The model under review builds one solid part; all positions refer to its coordinate system, in mm. Face numbers are marked on the shaded views. Round coordinates to 2 decimals unless told otherwise and drop trailing zeros. Loops run counter-clockwise (first coordinate to the right, second up) from the corner with the lowest first, then second, coordinate; pieces in that order, holes last. Notation, with made-up numbers: (-16.75, -27.5) -> (-7.75, -27.5) arc R24 cw to (-7.75, 0.5) -> close; hole circle Ø9 at (67.5, 84). An arc over 180 degrees is marked (long way). Return JSON: item names as keys, results as strings. Group by question number.
```python
from build123d import *

# Parameters (mm, degrees)
SKETCH_1_W          = 30
SKETCH_1_H          = 30
SKETCH_1_W_2        = 24
SKETCH_1_H_2        = 24
EXTRUDE_1_DEPTH     = 320
CUT_EXTRUDE_1_DEPTH = 323.800247831
SKETCH_3_R          = 2.1
CUT_EXTRUDE_2_DEPTH = 323.800247831
CUT_EXTRUDE_4_DEPTH = 323.800247831


with BuildPart() as part:
    # 草图1 → 拉伸-薄壁1 (new body)
    with BuildSketch(Plane.XY):
        with Locations((15, 15)):
            Rectangle(SKETCH_1_W, SKETCH_1_H)
        with Locations((15, 15)):
            Rectangle(SKETCH_1_W_2, SKETCH_1_H_2, mode=Mode.SUBTRACT)
    extrude(amount=EXTRUDE_1_DEPTH)

    # 草图2 → 切除-拉伸1 (cut, through all)
    with BuildSketch(Plane(origin=(30, 0, 0), x_dir=(0, 0, -1), z_dir=(1, 0, 0))):
        with BuildLine():
            Line((-277.5, 25), (-207.5, 25))
            ThreePointArc((-207.5, 25), (-197.5, 15), (-207.5, 5))
            Line((-207.5, 5), (-277.5, 5))
            ThreePointArc((-277.5, 5), (-287.5, 15), (-277.5, 25))
        make_face()
    extrude(amount=-CUT_EXTRUDE_1_DEPTH, mode=Mode.SUBTRACT)

    # 草图3 → 切除-拉伸2 (cut, through all)
    with BuildSketch(Plane(origin=(0, 30, 0), x_dir=(1, 0, 0), z_dir=(0, 1, 0))):
        with Locations(Location((15, -20, 0), (0, 0, 270))):
            Circle(SKETCH_3_R)
        with Locations(Location((15, -55, 0), (0, 0, 270))):
            Circle(SKETCH_3_R)
        with Locations(Location((15, -90, 0), (0, 0, 270))):
            Circle(SKETCH_3_R)
        with Locations(Location((15, -125, 0), (0, 0, 270))):
            Circle(SKETCH_3_R)
        with Locations(Location((15, -300, 0), (0, 0, 90))):
            Circle(SKETCH_3_R)
        with Locations(Location((15, -265, 0), (0, 0, 90))):
            Circle(SKETCH_3_R)
        with Locations(Location((15, -230, 0), (0, 0, 90))):
            Circle(SKETCH_3_R)
        with Locations(Location((15, -195, 0), (0, 0, 90))):
            Circle(SKETCH_3_R)
        with Locations(Location((15, -160, 0), (0, 0, 270))):
            Circle(SKETCH_3_R)
    extrude(amount=-CUT_EXTRUDE_2_DEPTH, mode=Mode.SUBTRACT)

    # 草图4 → 切除-拉伸4 (cut, through all)
    with BuildSketch(Plane(origin=(0, 0, 0), x_dir=(0, 0, -1), z_dir=(1, 0, 0))):
        Polygon((-180, 30), (-140, 3), (-80, 3), (-65, 30), align=None)
    extrude(amount=CUT_EXTRUDE_4_DEPTH, mode=Mode.SUBTRACT)


solid = part.part
```
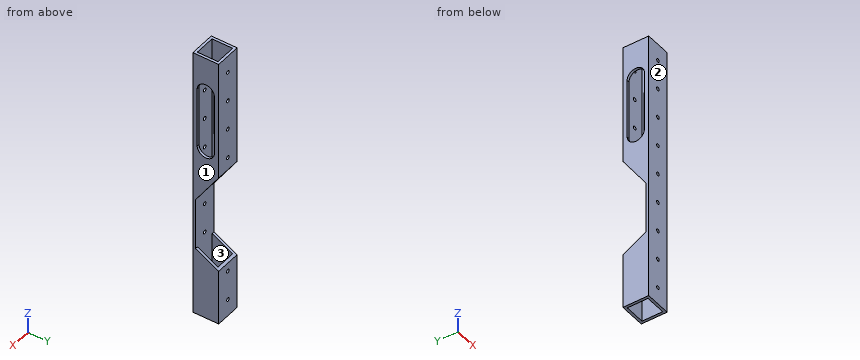
1. For P1, Ø6.5, axis at x = 15, z = 160, coming from the +Y side; P2, Ø5, axis at x = 15, z = 195, coming from the -Y side; P3, Ø2.5, axis at x = 15, z = 265, coming from the -Y side, all flat-tipped, find the tip position at first contact; note any pin that passes through.
2. Draft analysis for pull direction X (two halves, no side actions). For the marked faces 1, 2 and 3, state which applies: pulls with the +X half, pulls with the -X half, needs draft (parallel to the pull), parting line crosses it, or undercut.
3. We need section B-B, the plane z = 257. Write out the cut boundary in (x, y), then the cut area to 3 significant figures.
4. Wall thickness on line 1 (Y direction, x = 22, z = 291); line 2 (X direction, y = 28.1, z = 195): over which ranges is each line inside the solid? List them lowest first.
5. We need section A-A, the plane x = 21. Write out the cut boundary in (y, z).
6. We need section D-D, the plane z = 36.5. Write out the cut boundary in (x, y).
7. We need section C-C, the plane y = 22. Write out the cut boundary in (x, z), then the cut area to 3 significant figures.
Check sheet entries:
{
 "1": {"P1": "stops at y = 3", "P2": "stops at y = 0", "P3": "passes through"},
 "2": {"face 1": "pulls with the +X half", "face 2": "needs draft", "face 3": "undercut"},
 "3": {"outline": "(0, 0) -> (30, 0) -> (30, 5) -> (27, 5) -> (27, 3) -> (3, 3) -> (3, 5) -> (0, 5) -> close; (0, 25) -> (3, 25) -> (3, 27) -> (27, 27) -> (27, 25) -> (30, 25) -> (30, 30) -> (0, 30) -> close", "area": "204 mm²"},
 "4": {"line 1": "y = 0 to 3, 27 to 30", "line 2": "x = 0 to 12.9, 17.1 to 30"},
 "5": {"outline": "(0, 0) -> (3, 0) -> (3, 320) -> (0, 320) -> close; (27, 0) -> (30, 0) -> (30, 65) -> (27, 66.67) -> close; (27, 175.56) -> (30, 180) -> (30, 320) -> (27, 320) -> close"},
 "6": {"outline": "(0, 0) -> (30, 0) -> (30, 30) -> (0, 30) -> close; hole (3, 3) -> (27, 3) -> (27, 27) -> (3, 27) -> close"},
 "7": {"outline": "(0, 0) -> (3, 0) -> (3, 69.44) -> (0, 69.44) -> close; (0, 168.15) -> (3, 168.15) -> (3, 200.36) -> (0, 200.36) -> close; (0, 284.64) -> (3, 284.64) -> (3, 320) -> (0, 320) -> close; (27, 0) -> (30, 0) -> (30, 69.44) -> (27, 69.44) -> close; (27, 168.15) -> (30, 168.15) -> (30, 200.36) -> (27, 200.36) -> close; (27, 284.64) -> (30, 284.64) -> (30, 320) -> (27, 320) -> close", "area": "822 mm²"}
}
